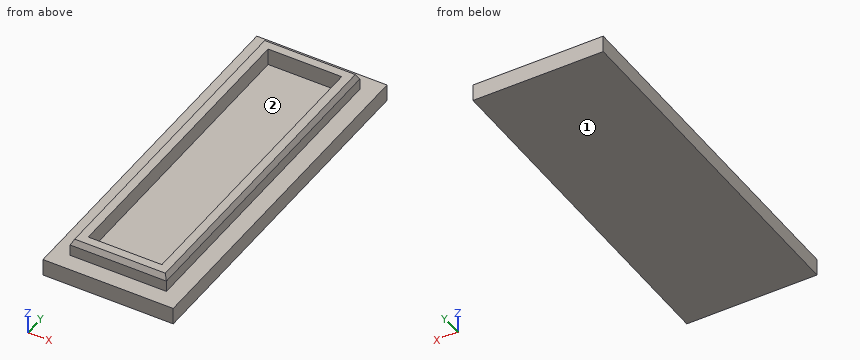
```python
from build123d import *

# Parameters (mm, degrees)
F0_W     = 23
F0_H     = 63
F1_DEPTH = 3
F2_W     = 17
F2_H     = 57
F2_W_2   = 13
F2_H_2   = 53
F3_DEPTH = 6
F4_SIZE2 = 0.5
F4_SIZE  = 1


with BuildPart() as f1:
    # F0 (on Top) → F1 (new body)
    with BuildSketch(Plane.XY):
        with Locations((11.5, 31.5)):
            Rectangle(F0_W, F0_H)
    extrude(amount=F1_DEPTH)

    # F2 (on face) → F3 (join)
    with BuildSketch(Plane(origin=(0, 0, 0), x_dir=(1, 0, 0), z_dir=(0, 0, -1))):
        with Locations((11.5, -31.5)):
            Rectangle(F2_W, F2_H)
        with Locations((11.5, -31.5)):
            Rectangle(F2_W_2, F2_H_2, mode=Mode.SUBTRACT)
    extrude(amount=-F3_DEPTH)

    # F4
    f4_edges = [f1.edges().sort_by_distance(p)[0] for p in [
        (11.5, 3, 6),
        (20, 31.5, 6),
        (3, 31.5, 6),
        (11.5, 60, 6),
    ]]
    chamfer(f4_edges, length=F4_SIZE, length2=F4_SIZE2)


solid = f1.part
```
The model under review builds one solid part; all positions refer to its coordinate system, in mm. Face numbers are marked on the shaded views. Give positions to 0.01 mm unless a question says otherwise; leave off trailing zeros. Write each loop counter-clockwise with the first axis right and the second up, starting at its lowest first coordinate (ties: lowest second). Pieces come first, ordered by that corner, then holes.
(1) Consider section C-C, the plane x = 2.25. Give the boundary of the cut face in (y, z).
(2) The part is to be moulded in two halves that separate along Y. For the marked faces 1 and 2, say which applies: released by +Y, released by -Y, zero draft, split by the parting line, or undercut.
(3) Consider section B-B, the plane x = 8.25. Give the boundary of the cut face in (y, z), and give its area (4 significant figures).
(4) For P1, Ø1.6, axis at y = 31, z = 4, coming from the +X side; P2, Ø0.6, axis at x = 12, z = 3.5, coming from the -Y side; P3, Ø2.5, axis at x = 8.5, z = 4, coming from the -Y side; P4, Ø0.6, axis at y = 40.5, z = 3.5, coming from the -X side, all flat-tipped, find the tip position at first contact; note any pin that passes through.
(5) Consider section A-A, the plane y = 17.5. Give the boundary of the cut face in (x, z).
(6) To check wall thickness, follow L1, parallel to X at y = 32, z = 4.25; L2, parallel to Z at x = 17.25, y = 34.5; L3, parallel to Y at x = 7.75, z = 4.25. State the ranges of each line that lie inside material, in increasing order.
Returned:
1. outline: (0, 0) - (63, 0) - (63, 3) - (0, 3) - close
2. face 1: zero draft
2. face 2: undercut
3. outline: (0, 0) - (63, 0) - (63, 3) - (60, 3) - (60, 5) - (59.5, 6) - (58, 6) - (58, 3) - (5, 3) - (5, 6) - (3.5, 6) - (3, 5) - (3, 3) - (0, 3) - close
3. area: 200.5 mm2
4. P1: stops at x = 20
4. P2: stops at y = 3
4. P3: stops at y = 0
4. P4: stops at x = 3
5. outline: (0, 0) - (23, 0) - (23, 3) - (20, 3) - (20, 5) - (19.5, 6) - (18, 6) - (18, 3) - (5, 3) - (5, 6) - (3.5, 6) - (3, 5) - (3, 3) - (0, 3) - close
6. L1: x = 3 to 5, 18 to 20
6. L2: z = 0 to 3
6. L3: y = 3 to 5, 58 to 60
